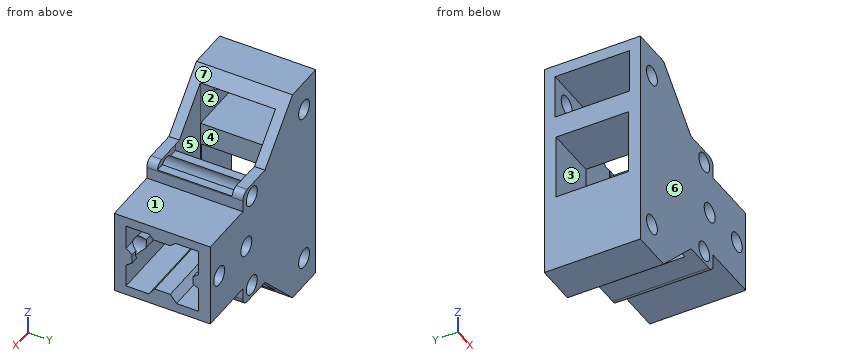
from build123d import *

# Parameters (mm, degrees)
F0_R      = 2.5
F1_DEPTH  = 12.5
F3_DEPTH  = 48.2856712694
F5_DEPTH  = 20
F7_DEPTH  = 50
F8_W      = 19.4369778037
F8_H      = 11.6137964651
F9_DEPTH  = 38.9448867569
F10_R     = 2.5
F11_DEPTH = 25.001


with BuildPart() as f1:
    # F0 (on Front) → F1 (new body, symmetric)
    with BuildSketch(Plane.XZ):
        with BuildLine():
            Line((9.3407845125, 0), (9.3407845125, 11.0652372241))
            Line((9.3407845125, 11.0652372241), (-5.5694617331, 11.0652372241))
            Line((-5.5694617331, 11.0652372241), (-5.5694617331, 14.1311359399))
            ThreePointArc((-5.5694617331, 14.1311359399), (-6.1552481707, 15.5453495022), (-7.5694617331, 16.1311359399))
            Line((-7.5694617331, 16.1311359399), (-15.6829056582, 16.1311359399))
            Line((-15.6829056582, 16.1311359399), (-28.3097643405, 29.1719902307))
            Line((-28.3097643405, 29.1719902307), (-38.9438867569, 29.1719902307))
            Line((-38.9438867569, 29.1719902307), (-38.9438867569, 0))
            Line((-38.9438867569, 0), (-38.9438867569, -29.1719902307))
            Line((-38.9438867569, -29.1719902307), (-28.3097643405, -29.1719902307))
            Line((-28.3097643405, -29.1719902307), (-15.6829056582, -16.1311359399))
            Line((-15.6829056582, -16.1311359399), (-7.5694617331, -16.1311359399))
            ThreePointArc((-7.5694617331, -16.1311359399), (-6.1552481707, -15.5453495022), (-5.5694617331, -14.1311359399))
            Line((-5.5694617331, -14.1311359399), (-5.5694617331, -11.0652372241))
            Line((-5.5694617331, -11.0652372241), (9.3407845125, -11.0652372241))
            Line((9.3407845125, -11.0652372241), (9.3407845125, 0))
        make_face()
        with Locations((-33.6268255487, -21.3849581778)):
            Circle(F0_R, mode=Mode.SUBTRACT)
        with Locations((-9.6699748597, -12.7693467682)):
            Circle(F0_R, mode=Mode.SUBTRACT)
        with Locations((-33.6268255487, 21.3849581778)):
            Circle(F0_R, mode=Mode.SUBTRACT)
        with Locations((-9.6699748597, 12.7693467682)):
            Circle(F0_R, mode=Mode.SUBTRACT)
    extrude(amount=F1_DEPTH, both=True)

    # F2 (on face) → F3 (cut, through all)
    with BuildSketch(Plane.YZ.offset(9.3407845125)):
        Polygon((9.4194319099, 8.595071733), (0, 8.595071733), (-9.4194319099, 8.595071733), (-9.4194319099, 0), (-9.4194319099, -8.595071733), (0, -8.595071733), (9.4194319099, -8.595071733), (9.4194319099, 0), align=None)
    extrude(amount=-F3_DEPTH, mode=Mode.SUBTRACT)

    # F4 (on face) → F5 (join)
    with BuildSketch(Plane.YZ.offset(9.3407845125)):
        Polygon((3.4560158383, 8.595071733), (-3.3186981454, 8.595071733), (-2.3508819286, 7.3865675367), (2.0042911638, 7.3865675367), align=None)
        Polygon((9.4194319099, -2.1302928217), (9.4194319099, 1.9829263911), (7.9856240889, 0.7893372769), (7.9856240889, -1.2431278592), align=None)
        Polygon((-1.9476253074, -6.5661179833), (-3.4800015856, -8.595071733), (3.6979699507, -8.595071733), (2.0849425346, -6.5661179833), align=None)
        Polygon((-7.8351749107, 0.9344584541), (-9.4194319099, 2.2248802707), (-9.4194319099, -2.6142010465), (-7.8351749107, -1.4044306008), align=None)
    extrude(amount=-F5_DEPTH)

    # F6 (on Top) → F7 (cut, symmetric)
    with BuildSketch(Plane.XY):
        Polygon((-13.8051696122, 9.7849667072), (-25.3022368997, 9.7849667072), (-25.3022368997, 0), (-25.3022368997, -9.7849667072), (-13.8051696122, -9.7849667072), (-13.8051696122, 0), align=None)
    extrude(amount=F7_DEPTH, both=True, mode=Mode.SUBTRACT)

    # F8 (on Right) → F9 (cut, through all)
    with BuildSketch(Plane.YZ):
        with Locations((-0.0271862373, 20.2530925162)):
            Rectangle(F8_W, F8_H)
    extrude(amount=-F9_DEPTH, mode=Mode.SUBTRACT)

    # F10 (on face) → F11 (cut, through all)
    with BuildSketch(Plane.XZ.offset(12.5)):
        with Locations((-7.1705817245, 0)):
            Circle(F10_R)
        with Locations((5.2617667243, 0)):
            Circle(F10_R)
    extrude(amount=-F11_DEPTH, mode=Mode.SUBTRACT)


solid = f1.part
Model file for the job. Use its own axes, mm. Face numbers are marked on the shaded views. A direction names the side the tool comes from. Round coordinates to 2 decimals unless told otherwise and drop trailing zeros. Loops run counter-clockwise (first coordinate to the right, second up) from the corner with the lowest first, then second, coordinate; pieces in that order, holes last. Notation, with made-up numbers: M -32,17 L 13,17 A24 cw 13,53 Z; hole C -23,25 d4. An arc over 180 degrees is marked long. One line per question, with ' | ' between items.
1) 3-axis set-ups, long thin cutter, end or side, ignore diameter. For the marked faces 1, 2, 3 and 4: which of +Z, -Z, +X, -X, +Y, -Y reach the whole face in a straight line?
Solved:
face 1: +Z, +X, +Y, -Y | face 2: +X, -X | face 3: -X | face 4: +Z, -Z
2) Band-saw the part on C-C (z = 0). Give the number of separate pieces and of enclosed holes in the cut face, then the cut area to 3 significant figures.
Solved:
separate pieces: 6 | enclosed holes: 0 | area: 258 mm²
3) Flat gauge pins, fed straight in: pin 1 (2 mm diameter, centred on x = -13.5, y = -10.5, fed in from +Z); pin 2 (12 mm diameter, centred on y = -3.5, z = 16, fed in from -X); pin 3 (2.5 mm diameter, centred on x = -12.5, y = 3.5, fed in from +Z); pin 4 (6 mm diameter, centred on y = -4.5, z = 20, fed in from +X). Where does each tip first touch, or does it go through?
Solved:
pin 1: stops at z = 16.13 | pin 2: stops at x = -38.94 | pin 3: stops at z = 14.45 | pin 4: passes through
4) Band-saw the part on A-A (x = -30). Give the cut face in (y, z), then the cut area to 3 significant figures.
Solved:
outline: M -12.5,-29.17 L 12.5,-29.17 L 12.5,29.17 L -12.5,29.17 Z; hole M -9.75,14.45 L 9.69,14.45 L 9.69,26.06 L -9.75,26.06 Z; hole M -9.42,-8.6 L 9.42,-8.6 L 9.42,8.6 L -9.42,8.6 Z | area: 909 mm²
5) Band-saw the part on D-D (z = -18). Give the cut face in (x, y), then the cut area to 3 significant figures.
Solved:
outline: M -38.94,-12.5 L -17.49,-12.5 L -17.49,-9.78 L -25.3,-9.78 L -25.3,9.78 L -17.49,9.78 L -17.49,12.5 L -38.94,12.5 Z | area: 383 mm²
6) Drill centre lines: line 1 along Z through (x, y) = (-30.5, 7); line 2 along X through (y, z) = (-4, 9); line 3 along Y through (x, z) = (1.5, -6.5). Where is each one in solid material? Low to high.
Solved:
line 1: z = -29.17 to -8.6, 8.6 to 14.45, 26.06 to 29.17 | line 2: x = -38.94 to -25.3, -13.81 to 9.34 | line 3: y = -12.5 to -9.42, 9.42 to 12.5
7) Mould opens along Y. For the marked faces 5, 6 and 7 say: +Y half, -Y half, draft (parallel to the pull), parting line (faces both ways), or undercut.
Solved:
face 5: undercut | face 6: -Y half | face 7: draft
8) Band-saw the part on B-B (x = -16.5). Give the cut face in (y, z).
Solved:
outline: M -12.5,-16.98 L -9.78,-16.98 L -9.78,16.98 L -12.5,16.98 Z; M 9.78,-16.98 L 12.5,-16.98 L 12.5,16.98 L 9.78,16.98 Z
